Verification items for the finished model (mm, model axes). A direction names the side the tool comes from. Round coordinates to 2 decimals unless told otherwise and drop trailing zeros. Loops run counter-clockwise (first coordinate to the right, second up) from the corner with the lowest first, then second, coordinate; pieces in that order, holes last. Notation, with made-up numbers: (-27, 68.5) -> (7, 68.5) arc R25 ccw to (7, 96.5) -> close; hole circle Ø9 at (21, 62.5). An arc over 180 degrees is marked (long way). Write item = value, one per line.
```python
from build123d import *
from build123d.topology import SkipClean

# Parameters (mm, degrees)
BOSS_EXTRUDE1_DEPTH      = 6
BOSS_EXTRUDE1_DEPTH_BACK = 4
SKETCH1_W                = 100
SKETCH1_H                = 50
SKETCH2_R                = 4.75
CUT_EXTRUDE1_DEPTH       = 57.789083458
MOVE_FACE2_BY            = 15
SKETCH3_W                = 100
SKETCH3_H                = 12
BOSS_EXTRUDE2_DEPTH      = 70
SKETCH4_R                = 2.5
BOSS_EXTRUDE3_DEPTH      = 20
SKETCH5_W                = 100
SKETCH5_H                = 56.133601368
BOSS_EXTRUDE4_DEPTH      = 10
CUT_EXTRUDE2_START       = -10
SKETCH6_R                = 4.75
SKETCH6_R_2              = 2.5
CUT_EXTRUDE2_DEPTH       = 10
FILLET2_R                = 24.5
FILLET3_R                = 5
CUT_EXTRUDE3_START       = -10
CUT_EXTRUDE3_DEPTH       = 10
BOSS_EXTRUDE5_START      = -10
SKETCH8_R                = 2.5
BOSS_EXTRUDE5_DEPTH      = 10
MOVE_START               = -4
MOVE_FACE3_DEPTH         = 10
SKETCH11_R               = 7.5
BOSS_EXTRUDE6_DEPTH      = 70
CUT_EXTRUDE4_START       = -70
CUT_EXTRUDE4_DEPTH       = 70
SKETCH13_R               = 3.5
CUT_EXTRUDE5_DEPTH       = 103.46950766
MOVE_START_2             = 6
MOVE_FACE4_OUTLINE_R     = 7.5
MOVE_FACE4_OUTLINE_R_2   = 3.5
MOVE_FACE4_DEPTH         = 70
MOVE_FACE4_2_OUTLINE_R   = 7.5
MOVE_FACE4_2_OUTLINE_R_2 = 3.5
MOVE_FACE4_2_DEPTH       = 80
MOVE_FACE4_3_OUTLINE_R   = 3.5
MOVE_FACE4_3_DEPTH       = 10
MOVE_FACE5_DEPTH         = 10
MOVE_FACE5_2_DEPTH       = 10
MOVE_FACE6_DEPTH         = 10
SKETCH17_R               = 3.5
CUT_EXTRUDE9_DEPTH       = 10


# Read off the part's stored shape, not the designer's step: Move Face3, Move Face4, Move Face5, Move Face6
with BuildPart() as part:
    # Sketch1 → Boss-Extrude1 (new, two sides: drawn at the far end of the back side and taken through both)
    with BuildSketch(Plane.XY.offset(-BOSS_EXTRUDE1_DEPTH_BACK)):
        Rectangle(SKETCH1_W, SKETCH1_H)
    extrude(amount=BOSS_EXTRUDE1_DEPTH + BOSS_EXTRUDE1_DEPTH_BACK)

    # Sketch2 → Cut-Extrude1 (cut, through all)
    with BuildSketch(Plane.XY.offset(6)):
        with Locations((27.75, 0)):
            Circle(SKETCH2_R)
        with Locations((-27.75, 0)):
            Circle(SKETCH2_R)
    extrude(amount=-CUT_EXTRUDE1_DEPTH, mode=Mode.SUBTRACT)

    # Move Face2: a face moved outward by 15.0
    extrude(part.faces().sort_by_distance((0, 25, 1))[0], amount=MOVE_FACE2_BY, dir=(0, 1, 0))

    # Sketch3 → Boss-Extrude2 (add)
    with BuildSketch(Plane.XY.offset(6)):
        with Locations((0, 34)):
            Rectangle(SKETCH3_W, SKETCH3_H)
    extrude(amount=BOSS_EXTRUDE2_DEPTH)

    # Sketch4 → Boss-Extrude3 (add)
    with BuildSketch(Plane(origin=(0, 0, -4), x_dir=(-1, 0, 0), z_dir=(0, 0, -1))):
        with Locations((9.999238357, -11.441146597)):
            Circle(SKETCH4_R)
        with Locations((-10.000761643, -9.892069005)):
            Circle(SKETCH4_R)
    extrude(amount=-BOSS_EXTRUDE3_DEPTH)

    # Sketch5 → Boss-Extrude4 (add)
    with BuildSketch(Plane.XY.offset(76)):
        with Locations((0, 11.933199316)):
            Rectangle(SKETCH5_W, SKETCH5_H)
    extrude(amount=BOSS_EXTRUDE4_DEPTH)

    # Sketch6 → Cut-Extrude2 (cut)
    with BuildSketch(Plane(origin=(0, 0, -4), x_dir=(-1, 0, 0), z_dir=(0, 0, -1)).offset(CUT_EXTRUDE2_START)):
        with Locations(Location((27.75, 0, 0), (0, 0, 180))):
            Circle(SKETCH6_R)
        with Locations((10.004296788, -9.901140623)):
            Circle(SKETCH6_R_2)
        with Locations((-9.995700599, -9.91136318)):
            Circle(SKETCH6_R_2)
        with Locations(Location((-27.75, 0, 0), (0, 0, 180))):
            Circle(SKETCH6_R)
    extrude(amount=CUT_EXTRUDE2_DEPTH, mode=Mode.SUBTRACT)

    # Fillet2
    # the kernel refuses this fillet: 24.5 mm, written as the material it takes off along each edge
    with BuildSketch(Plane(origin=(50, -16.133601368, 14.75), x_dir=(0, 1, 0), z_dir=(0, 0, 1)), Plane(origin=(50, -25, -65.25), x_dir=(0, 1, 0), z_dir=(0, 0, 1))) as fillet2_piece_1:
        with BuildLine():
            CenterArc((FILLET2_R, FILLET2_R), FILLET2_R, 180, 90)
            Line((0, FILLET2_R), (0, 0))
            Line((0, 0), (FILLET2_R, 0))
        make_face()
    extrude(amount=132.5, mode=Mode.SUBTRACT)
    with BuildSketch(Plane(origin=(-50, 40, 147.25), x_dir=(0, -1, 0), z_dir=(0, 0, -1)), Plane(origin=(50, 40, -65.25), x_dir=(0, -1, 0), z_dir=(0, 0, 1))) as fillet2_piece_2:
        with BuildLine():
            CenterArc((FILLET2_R, -FILLET2_R), FILLET2_R, 90, 90)
            Line((0, -FILLET2_R), (0, 0))
            Line((0, 0), (FILLET2_R, 0))
        make_face()
    extrude(amount=212.5, mode=Mode.SUBTRACT)
    with BuildSketch(Plane(origin=(-50, -16.133601368, 14.75), x_dir=(0, 1, 0), z_dir=(0, 0, 1)), Plane(origin=(-50, -25, 67.25), x_dir=(1, 0, 0), z_dir=(0, 0, -1))) as fillet2_piece_3:
        with BuildLine():
            CenterArc((FILLET2_R, -FILLET2_R), FILLET2_R, 90, 90)
            Line((0, -FILLET2_R), (0, 0))
            Line((0, 0), (FILLET2_R, 0))
        make_face()
    extrude(amount=132.5, mode=Mode.SUBTRACT)

    # Fillet3
    fillet3_edges = [part.edges().sort_by_distance(p)[0] for p in [
        (46.571307506, 28, 41),
        (-46.571307506, 28, 41),
    ]]
    fillet(fillet3_edges, radius=FILLET3_R)

    # Sketch7 → Cut-Extrude3 (cut)
    with BuildSketch(Plane.XY.offset(86).offset(CUT_EXTRUDE3_START)):
        with BuildLine():
            Line((-25.5, -16.133601368), (25.5, -16.133601368))
            ThreePointArc((25.5, -16.133601368), (42.824116139, -8.957717507), (50, 8.366398632))
            Line((50, 8.366398632), (50, 15.5))
            ThreePointArc((50, 15.5), (42.824116139, 32.824116139), (25.5, 40))
            Line((25.5, 40), (-25.5, 40))
            ThreePointArc((-25.5, 40), (-42.824116139, 32.824116139), (-50, 15.5))
            Line((-50, 15.5), (-50, 8.366398632))
            ThreePointArc((-50, 8.366398632), (-42.824116139, -8.957717507), (-25.5, -16.133601368))
        make_face()
    extrude(amount=CUT_EXTRUDE3_DEPTH, mode=Mode.SUBTRACT)

    # Sketch8 → Boss-Extrude5 (add)
    with BuildSketch(Plane(origin=(0, 0, -4), x_dir=(-1, 0, 0), z_dir=(0, 0, -1)).offset(BOSS_EXTRUDE5_START)):
        with Locations((10.004296788, -9.901140623)):
            Circle(SKETCH8_R)
        with Locations((-9.995700599, -9.91136318)):
            Circle(SKETCH8_R)
    extrude(amount=BOSS_EXTRUDE5_DEPTH)

    # Move Face3 outline → Move Face3 (cut)
    with BuildSketch(Plane.XY.offset(MOVE_START)):
        with BuildLine():
            Line((25.5, -20), (-25.5, -20))
            ThreePointArc((-25.5, -20), (-42.824116139, -12.824116139), (-50, 4.5))
            Line((-50, 4.5), (-50, -0.5))
            ThreePointArc((-50, -0.5), (-42.824116139, -17.824116139), (-25.5, -25))
            Line((-25.5, -25), (25.5, -25))
            ThreePointArc((25.5, -25), (42.824116139, -17.824116139), (50, -0.5))
            Line((50, -0.5), (50, 4.5))
            ThreePointArc((50, 4.5), (42.824116139, -12.824116139), (25.5, -20))
        make_face()
    extrude(amount=MOVE_FACE3_DEPTH, mode=Mode.SUBTRACT)

    # Sketch11 → Boss-Extrude6 (add)
    with BuildSketch(Plane.XY.offset(6)):
        with Locations((-20, 28.450922409)):
            Circle(SKETCH11_R)
        with Locations((20, 28.450922409)):
            Circle(SKETCH11_R)
    extrude(amount=BOSS_EXTRUDE6_DEPTH)

    # Sketch12 → Cut-Extrude4 (cut)
    with SkipClean():  # the faces are left unmerged after this step: merging them gives an invalid solid
        with BuildSketch(Plane.XY.offset(76).offset(CUT_EXTRUDE4_START)):
            with BuildLine():
                Line((-34.102325267, 28), (-27.486432327, 28))
                ThreePointArc((-27.486432327, 28), (-20, 35.950922409), (-12.513567673, 28))
                Line((-12.513567673, 28), (12.513567673, 28))
                ThreePointArc((12.513567673, 28), (20, 35.950922409), (27.486432327, 28))
                Line((27.486432327, 28), (34.102325267, 28))
                ThreePointArc((34.102325267, 28), (38.972432937, 31.867722966), (36.308049694, 37.487179487))
                ThreePointArc((36.308049694, 37.487179487), (31.048157467, 39.363527583), (25.5, 40))
                Line((25.5, 40), (-25.5, 40))
                ThreePointArc((-25.5, 40), (-31.048157467, 39.363527583), (-36.308049694, 37.487179487))
                ThreePointArc((-36.308049694, 37.487179487), (-38.972432937, 31.867722966), (-34.102325267, 28))
            make_face()
        extrude(amount=CUT_EXTRUDE4_DEPTH, mode=Mode.SUBTRACT)

    # Sketch13 → Cut-Extrude5 (cut, through all)
    with SkipClean():  # the faces are left unmerged after this step: merging them gives an invalid solid
        with BuildSketch(Plane.XY.offset(76)):
            with Locations((-20, 28.450922409)):
                Circle(SKETCH13_R)
            with Locations((20, 28.450922409)):
                Circle(SKETCH13_R)
        extrude(amount=-CUT_EXTRUDE5_DEPTH, mode=Mode.SUBTRACT)

    # Move Face4 outline → Move Face4 (cut)
    # profile 1 of 2: a face of its own
    with BuildSketch(Plane.XY.offset(MOVE_START_2)):
        with Locations((20, 28.450922409)):
            Circle(MOVE_FACE4_OUTLINE_R)
        with Locations((20, 28.450922409)):
            Circle(MOVE_FACE4_OUTLINE_R_2, mode=Mode.SUBTRACT)
    # profile 2 of 2: a face of its own
    with BuildSketch(Plane.XY.offset(MOVE_START_2)):
        with Locations((-20, 28.450922409)):
            Circle(MOVE_FACE4_OUTLINE_R)
        with Locations((-20, 28.450922409)):
            Circle(MOVE_FACE4_OUTLINE_R_2, mode=Mode.SUBTRACT)
    extrude(amount=MOVE_FACE4_DEPTH, mode=Mode.SUBTRACT)

    # Move Face4 2 outline → Move Face4 2 (add)
    # profile 1 of 2: a face of its own
    with BuildSketch(Plane.XY.offset(MOVE_START)):
        with Locations((20, 46.450922409)):
            Circle(MOVE_FACE4_2_OUTLINE_R)
        with Locations((20, 46.450922409)):
            Circle(MOVE_FACE4_2_OUTLINE_R_2, mode=Mode.SUBTRACT)
    # profile 2 of 2: a face of its own
    with BuildSketch(Plane.XY.offset(MOVE_START)):
        with Locations((-20, 46.450922409)):
            Circle(MOVE_FACE4_2_OUTLINE_R)
        with Locations((-20, 46.450922409)):
            Circle(MOVE_FACE4_2_OUTLINE_R_2, mode=Mode.SUBTRACT)
    extrude(amount=MOVE_FACE4_2_DEPTH)

    # Move Face4 3 outline → Move Face4 3 (add)
    with BuildSketch(Plane.XY.offset(MOVE_START)):
        with BuildLine():
            ThreePointArc((50, 33.5), (42.824116139, 50.824116139), (25.5, 58))
            Line((25.5, 58), (-25.5, 58))
            ThreePointArc((-25.5, 58), (-42.824116139, 50.824116139), (-50, 33.5))
            Line((-50, 33.5), (-50, 15.5))
            ThreePointArc((-50, 15.5), (-42.824116139, 32.824116139), (-25.5, 40))
            Line((-25.5, 40), (-23.825650281, 40))
            ThreePointArc((-23.825650281, 40), (-20, 53.950922409), (-16.174349719, 40))
            Line((-16.174349719, 40), (16.174349719, 40))
            ThreePointArc((16.174349719, 40), (20, 53.950922409), (23.825650281, 40))
            Line((23.825650281, 40), (25.5, 40))
            ThreePointArc((25.5, 40), (42.824116139, 32.824116139), (50, 15.5))
            Line((50, 15.5), (50, 33.5))
        make_face()
        with Locations((20, 28.450922409)):
            Circle(MOVE_FACE4_3_OUTLINE_R)
        with Locations((-20, 28.450922409)):
            Circle(MOVE_FACE4_3_OUTLINE_R)
    extrude(amount=MOVE_FACE4_3_DEPTH)

    # Move Face5 outline → Move Face5 (cut)
    with BuildSketch(Plane.XY.offset(MOVE_START)):
        with BuildLine():
            ThreePointArc((-32.436349859, -0.775), (-27.75, -6.3), (-23.063650141, -0.775))
            ThreePointArc((-23.063650141, -0.775), (-27.75, -4.75), (-32.436349859, -0.775))
        make_face()
        with BuildLine():
            ThreePointArc((23.063650141, -0.775), (27.75, -6.3), (32.436349859, -0.775))
            ThreePointArc((32.436349859, -0.775), (27.75, -4.75), (23.063650141, -0.775))
        make_face()
    extrude(amount=MOVE_FACE5_DEPTH, mode=Mode.SUBTRACT)

    # Move Face5 2 outline → Move Face5 2 (add)
    with BuildSketch(Plane.XY.offset(MOVE_START)):
        with BuildLine():
            ThreePointArc((-32.436349859, -0.775), (-27.75, 3.2), (-23.063650141, -0.775))
            ThreePointArc((-23.063650141, -0.775), (-27.75, 4.75), (-32.436349859, -0.775))
        make_face()
        with BuildLine():
            ThreePointArc((23.063650141, -0.775), (27.75, 3.2), (32.436349859, -0.775))
            ThreePointArc((32.436349859, -0.775), (27.75, 4.75), (23.063650141, -0.775))
        make_face()
    extrude(amount=MOVE_FACE5_2_DEPTH)

    # Move Face6 outline → Move Face6 (add)
    with BuildSketch(Plane.XY.offset(MOVE_START)):
        with BuildLine():
            ThreePointArc((50, 41.5), (42.824116139, 58.824116139), (25.5, 66))
            Line((25.5, 66), (-25.5, 66))
            ThreePointArc((-25.5, 66), (-42.824116139, 58.824116139), (-50, 41.5))
            Line((-50, 41.5), (-50, 33.5))
            ThreePointArc((-50, 33.5), (-42.824116139, 50.824116139), (-25.5, 58))
            Line((-25.5, 58), (25.5, 58))
            ThreePointArc((25.5, 58), (42.824116139, 50.824116139), (50, 33.5))
            Line((50, 33.5), (50, 41.5))
        make_face()
    extrude(amount=MOVE_FACE6_DEPTH)

    # Sketch17 → Cut-Extrude9 (cut)
    with BuildSketch(Plane(origin=(0, 0, -4), x_dir=(-1, 0, 0), z_dir=(0, 0, -1))):
        with Locations((-20, 26.450922409)):
            Circle(SKETCH17_R)
        with Locations((20, 26.450922409)):
            Circle(SKETCH17_R)
    extrude(amount=-CUT_EXTRUDE9_DEPTH, mode=Mode.SUBTRACT)


solid = part.part
```
(1) Sectioned sample at C-C, the plane y = 34.5. Record the cut outline in (x, z).
Filled sheet:
outline = (-50, -4) -> (50, -4) -> (50, 6) -> (-50, 6) -> close
(2) Set-up check for faces 4 (the face through (-18.38, 43.35, 35.44)), 5 (the face through (-8.16, -9.75, 10.93)): record each of +Z, -Z, +X, -X, +Y, -Y from which the full face is reachable in a straight line by a thin tool's end or side.
Filled sheet:
face_4 = +Z, -Z
face_5 = +Z
(3) Sectioned sample at D-D, the plane x = -9. Record the cut outline in (y, z), and give its area (3 significant figures).
Filled sheet:
outline = (-20, -4) -> (66, -4) -> (66, 6) -> (-9.15, 6) -> (-9.15, 16) -> (-13.73, 16) -> (-13.73, 6) -> (-20, 6) -> close
area = 906 mm2
(4) Draft check along X on faces 1 (the face through (-42.633, -13.014, 0.93)), 2 (the face through (21.62, 43.35, 35.44)), 3 (the face through (-1, 24, -4)). Enter one of: released by +X, released by -X, zero draft, split by the parting line, or undercut.
Filled sheet:
face_1 = released by -X
face_2 = undercut
face_3 = zero draft
(5) Sectioned sample at A-A, the plane x = 20. Record the cut outline in (y, z).
Filled sheet:
outline = (-20, -4) -> (22.95, -4) -> (22.95, 6) -> (-20, 6) -> close; (29.95, -4) -> (42.95, -4) -> (42.95, 76) -> (38.95, 76) -> (38.95, 6) -> (29.95, 6) -> close; (49.95, -4) -> (66, -4) -> (66, 6) -> (53.95, 6) -> (53.95, 76) -> (49.95, 76) -> close
(6) Sectioned sample at B-B, the plane z = 63. Record the cut outline in (x, y), and give its area (3 significant figures).
Filled sheet:
outline = circle Ø15 at (-20, 46.45); circle Ø15 at (20, 46.45); hole circle Ø7 at (-20, 46.45); hole circle Ø7 at (20, 46.45)
area = 276 mm2
(7) Go/stop test with flat-tipped pins: pin 1 Ø2.5 at (x, y) = (9.5, -9) entering from +Z; pin 2 Ø12 at (y, z) = (41, 27) entering from -X; pin 3 Ø6 at (x, z) = (-25.5, 19.5) entering from +Y. Record where each tip stops, or that it passes through.
Filled sheet:
pin_1 = 16
pin_2 = -27.5
pin_3 = 53.52
(8) Material ranges on probe 1 along X at (y, z) = (-1.55, -1.75); probe 2 along Y at (x, z) = (-20, 3); probe 3 along X at (y, z) = (45, 70), recorded low to high. Write a range as from..to.
Filled sheet:
probe_1 = -49.24..-32.5, -23..23, 32.5..49.24
probe_2 = -20..22.95, 29.95..42.95, 49.95..66
probe_3 = -27.36..-23.19, -16.81..-12.64, 12.64..16.81, 23.19..27.36
